Part print with two shaded views. Sizes in mm from the minimum x, y, z corner. Round coordinates to 2 decimals unless told otherwise and drop trailing zeros. Order: outer loops, then holes, each group sorted by start corner. A loop starts at its lowest first (then second) coordinate and runs counter-clockwise, first axis right, second up. Notation, with made-up numbers: (29, -9) -> (69, -9) arc R28 ccw to (69, 16) -> close; hole circle Ø7 at (26, 55). An arc over 180 degrees is marked (long way). Answer as a JSON object with one key per item and string values.
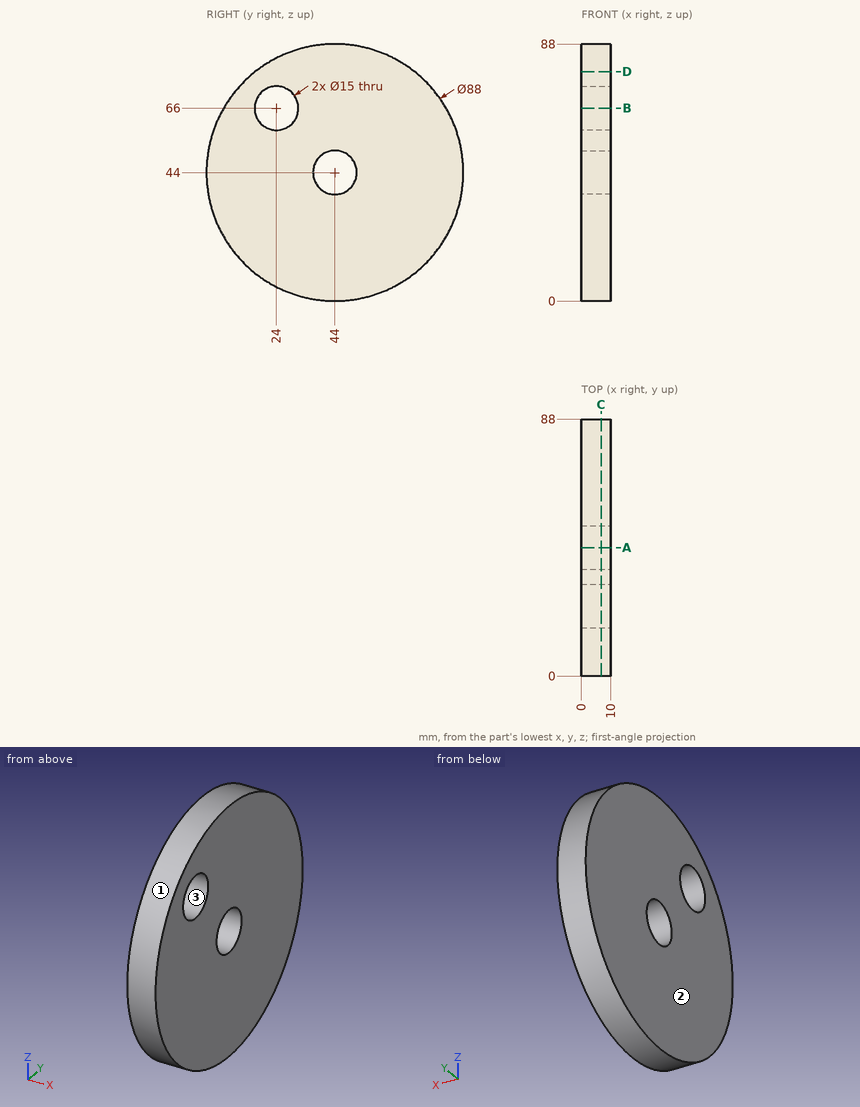
1) Pull direction Z, two halves, no side cores. Call the marked faces 1, 2 and 3: pulls with the +Z half, pulls with the -Z half, needs draft (parallel to the pull), parting line crosses it, or undercut.
Checked values:
{"face 1": "parting line crosses it", "face 2": "needs draft", "face 3": "undercut"}
2) Cut at D-D, the plane z = 78.5. Give the cut face in (x, y), plus the area to 3 significant figures.
Checked values:
{"outline": "(0, 16.69) -> (10, 16.69) -> (10, 71.31) -> (0, 71.31) -> close", "area": "546 mm²"}
3) Cut at B-B, the plane z = 66. Give the cut face in (x, y).
Checked values:
{"outline": "(0, 5.89) -> (10, 5.89) -> (10, 16.5) -> (0, 16.5) -> close; (0, 31.5) -> (10, 31.5) -> (10, 82.11) -> (0, 82.11) -> close"}
4) Cut at C-C, the plane x = 6.75. Give the cut face in (y, z), plus the area to 3 significant figures.
Checked values:
{"outline": "circle Ø88 at (44, 44); hole circle Ø15 at (24, 66); hole circle Ø15 at (44, 44)", "area": "5,730 mm²"}
5) Probe L1, parallel to Y at x = 4, z = 68.5; L2, parallel to Z at x = 3.5, y = 47.5; L3, parallel to Y at x = 6, z = 66. List the from-to ranges inside material, lowest first. Write a range as from..to.
Checked values:
{"L1": "y = 7.45..16.93, 31.07..80.55", "L2": "z = 0.14..37.37, 50.63..87.86", "L3": "y = 5.89..16.5, 31.5..82.11"}
6) Cut at A-A, the plane y = 44. Give the cut face in (x, z).
Checked values:
{"outline": "(0, 0) -> (10, 0) -> (10, 36.5) -> (0, 36.5) -> close; (0, 51.5) -> (10, 51.5) -> (10, 88) -> (0, 88) -> close"}
7) Flat gauge pins, fed straight in: pin 1 Ø1.5 at (x, y) = (3.5, 38.5) entering from +Z; pin 2 Ø5 at (x, z) = (5.5, 15.5) entering from +Y; pin 3 Ø9 at (y, z) = (44, 44) entering from +X. Where does each tip first touch, or does it go through?
Checked values:
{"pin 1": "stops at z = 87.74", "pin 2": "stops at y = 79.5", "pin 3": "passes through"}
